Read the model definition and answer for the solid it produces. Units are mm, in the model's axes. A direction names the side the tool comes from. Coordinates: 2 decimals unless noted, no trailing zeros. Order: outer loops, then holes, each group sorted by start corner. A loop starts at its lowest first (then second) coordinate and runs counter-clockwise, first axis right, second up. Notation, with made-up numbers: (5.5, 52.25) -> (9.5, 52.25) arc R28 cw to (9.5, 90.25) -> close; hole circle Ø4 at (72, 35). An arc over 180 degrees is marked (long way). Use CSV: the item, a comma, the result in double quotes.
```python
from build123d import *

# Parameters (mm, degrees)
SKETCH1_R           = 158
SKETCH1_R_2         = 123
SKETCH1_R_3         = 5.25
BOSS_EXTRUDE1_DEPTH = 10
SKETCH2_R           = 125
CUT_EXTRUDE1_DEPTH  = 3
CHAMFER1_SIZE       = 1


with BuildPart() as part:
    # Sketch1 → Boss-Extrude1 (new body)
    with BuildSketch(Plane(origin=(0, 0, 0), x_dir=(1, 0, 0), z_dir=(0, 1, 0))):
        Circle(SKETCH1_R)
        Circle(SKETCH1_R_2, mode=Mode.SUBTRACT)
        with Locations((0, 140.5)):
            Circle(SKETCH1_R_3, mode=Mode.SUBTRACT)
        with Locations((121.676569232, 70.25)):
            Circle(SKETCH1_R_3, mode=Mode.SUBTRACT)
        with Locations((121.676569232, -70.25)):
            Circle(SKETCH1_R_3, mode=Mode.SUBTRACT)
        with Locations((0, -140.5)):
            Circle(SKETCH1_R_3, mode=Mode.SUBTRACT)
        with Locations((-121.676569232, -70.25)):
            Circle(SKETCH1_R_3, mode=Mode.SUBTRACT)
        with Locations((-121.676569232, 70.25)):
            Circle(SKETCH1_R_3, mode=Mode.SUBTRACT)
    extrude(amount=BOSS_EXTRUDE1_DEPTH)

    # Sketch2 → Cut-Extrude1 (cut)
    with BuildSketch(Plane.XZ):
        Circle(SKETCH2_R)
    extrude(amount=-CUT_EXTRUDE1_DEPTH, mode=Mode.SUBTRACT)

    # Chamfer1
    chamfer1_edges = [part.edges().sort_by_distance(p)[0] for p in [
        (-125, 0, 0),
    ]]
    chamfer(chamfer1_edges, length=CHAMFER1_SIZE)


solid = part.part
```
Item 1: Find section A-A, the plane z = 0. Give the vertices of the cut face in (x, y).
Return value:
outline,"(-158, 0) -> (-126, 0) -> (-125, 1) -> (-125, 3) -> (-123, 3) -> (-123, 10) -> (-158, 10) -> close; (123, 3) -> (125, 3) -> (125, 1) -> (126, 0) -> (158, 0) -> (158, 10) -> (123, 10) -> close"
Item 2: Each of these flat-tipped pins is pushed along its axis until it touches: P1, Ø6, axis at y = 7.5, z = -91, coming from the +X side (3 decimals); P2, Ø5, axis at y = 4, z = -113.5, coming from the +X side. Where does it stop, or does it pass through?
Return value:
P1,"stops at x = 131.225"
P2,"stops at x = 112.44"
Item 3: The mould has two halves that part along X. Classify faces 1 (the cylindrical face through (-116.453, 4.93, -106.784)), 2 (the flat face through (-36, 10, -118)), 3 (the cylindrical face through (-116.67, 4.93, -71.83)): +X half, -X half, draft (parallel to the pull), parting line (faces both ways), or undercut.
Return value:
face 1,"parting line"
face 2,"draft"
face 3,"undercut"
Item 4: Find section C-C, the plane z = 70.25. Give the number of separate pieces and of enclosed holes in the cut face, then the cut area to 3 significant figures.
Return value:
separate pieces,"4"
enclosed holes,"0"
area,"585 mm^2"
Item 5: Straight lines are drawn through the part: line 1 along Z through (x, y) = (0, 2.35); line 2 along X through (y, z) = (6.5, 70.25); line 3 along Z through (x, y) = (0, 6.75). For each, find the intervals that lie inside material, in ascending order.
Return value:
line 1,"z = -158 to -145.75, -135.25 to -125, 125 to 135.25, 145.75 to 158"
line 2,"x = -141.52 to -126.93, -116.43 to -100.97, 100.97 to 116.43, 126.93 to 141.52"
line 3,"z = -158 to -145.75, -135.25 to -123, 123 to 135.25, 145.75 to 158"
Item 6: A tool of negligible diameter and unlimited length cuts with its end or side. For faces 4 (the flat face through (92, 3, -83)), 5 (the cylindrical face through (-1.138, 4.93, -135.375)), from which of +Z, -Z, +X, -X, +Y, -Y can it reach the whole face along a straight path? Write none if from no direction.
Return value:
face 4,"-Y"
face 5,"+Y, -Y"
Item 7: Find section B-B, the plane z = 140.5. Give the vertices of the cut face in (x, y).
Return value:
outline,"(-72.28, 0) -> (-5.25, 0) -> (-5.25, 10) -> (-72.28, 10) -> close; (5.25, 0) -> (72.28, 0) -> (72.28, 10) -> (5.25, 10) -> close"
